The listing builds one solid part. Answer for the finished solid, in the listing's coordinates (mm). Face numbers are marked on the shaded views. A direction names the side the tool comes from. Give positions to 0.01 mm unless a question says otherwise; leave off trailing zeros. Order: outer loops, then holes, each group sorted by start corner. A loop starts at its lowest first (then second) coordinate and runs counter-clockwise, first axis right, second up. Notation, with made-up numbers: (57.25, 56) - (91.25, 56) arc R28 cw to (91.25, 90) - close; hole circle Ø4 at (-1.75, 30). An arc over 180 degrees is marked (long way). Write each question's results on one line, items separated by ' | '. Start each with the question number.
1. Section A-A (x = 22) is taken. Give the vertices of the cut face in (y, z).
2. Flat-ended cylindrical pins translate along their axes: pin 1 (8 mm diameter, centred on x = 33.5, y = 11, fed in from +Z); pin 2 (18.5 mm diameter, centred on x = 0, z = 0, fed in from -Y); pin 3 (1 mm diameter, centred on y = 4.5, z = -13, fed in from -X). Find the tip coordinate at first contact, or state that the pin passes through.
3. Which of the six approach directions +Z, -Z, +X, -X, +Y, -Y give full straight-line access (tool end or side, diameter ignored) to the marked faces 5 and 6?
4. Find the intervals of material crossed by L1, parallel to Z at x = 22, y = 14.5; L2, parallel to X at y = 10, z = -6.75; L3, parallel to Z at x = 0.5, y = 13.5, in increasing order.
5. Section B-B (y = 10) is taken. Give the vertices of the cut face in (x, z).
6. Section C-C (x = 31.7) is taken. Give the vertices of the cut face in (y, z), and give its area (3 significant figures).
7. Determine the mould class of the marked faces 1, 2, 3 and 4 for opening direction Z: released by +Z, released by -Z, zero draft, split by the parting line, or undercut.
8. Section D-D (z = 0) is taken. Give the vertices of the cut face in (x, y), and give its area (3 significant figures).
from build123d import *

# Parameters (mm, degrees)
DODANIE_WYCI_GNI_CIE1_DEPTH  = 20
ZAAWANSOWANYOTW_R1_START     = -11.5
ZAAWANSOWANYOTW_R1_OUTLINE_R = 5.5
ZAAWANSOWANYOTW_R1_DEPTH     = 23
ZAOKR_GLENIE3_R              = 2


# Read off the part's stored shape, not the designer's step: ZaawansowanyOtwór1
with BuildPart() as part:
    # Szkic1 → Dodanie-wyciągnięcie1 (new body)
    with BuildSketch(Plane(origin=(0, 0, 0), x_dir=(1, 0, 0), z_dir=(0, 1, 0))):
        with BuildLine():
            Line((12.109500403, 11.5), (39.7, 11.5))
            ThreePointArc((39.7, 11.5), (41.114213562, 10.914213562), (41.7, 9.5))
            Line((41.7, 9.5), (41.7, 4.5))
            ThreePointArc((41.7, 4.5), (41.114213562, 3.085786438), (39.7, 2.5))
            Line((39.7, 2.5), (13.774977314, 2.5))
            Line((13.774977314, 2.5), (12.939860896, 2.5))
            ThreePointArc((12.939860896, 2.5), (11.780953784, 2.869989477), (11.050830108, 3.843065693))
            ThreePointArc((11.050830108, 3.843065693), (-11.7, 0), (11.050830108, -3.843065693))
            ThreePointArc((11.050830108, -3.843065693), (11.780953784, -2.869989477), (12.939860896, -2.5))
            Line((12.939860896, -2.5), (13.774977314, -2.5))
            Line((13.774977314, -2.5), (39.7, -2.5))
            ThreePointArc((39.7, -2.5), (41.114213562, -3.085786438), (41.7, -4.5))
            Line((41.7, -4.5), (41.7, -9.5))
            ThreePointArc((41.7, -9.5), (41.114213562, -10.914213562), (39.7, -11.5))
            Line((39.7, -11.5), (12.109500403, -11.5))
            ThreePointArc((12.109500403, -11.5), (-16.7, 0), (12.109500403, 11.5))
        make_face()
    extrude(amount=DODANIE_WYCI_GNI_CIE1_DEPTH)

    # ZaawansowanyOtwór1 outline → ZaawansowanyOtwór1 (cut)
    with BuildSketch(Plane.XY.offset(ZAAWANSOWANYOTW_R1_START)):
        with Locations((31.7, 10)):
            Circle(ZAAWANSOWANYOTW_R1_OUTLINE_R)
    extrude(amount=ZAAWANSOWANYOTW_R1_DEPTH, mode=Mode.SUBTRACT)

    # Zaokrąglenie3
    zaokr_glenie3_edges = [part.edges().sort_by_distance(p)[0] for p in [
        (-16.7, 0, 0),
        (-16.7, 20, 0),
    ]]
    fillet(zaokr_glenie3_edges, radius=ZAOKR_GLENIE3_R)


solid = part.part
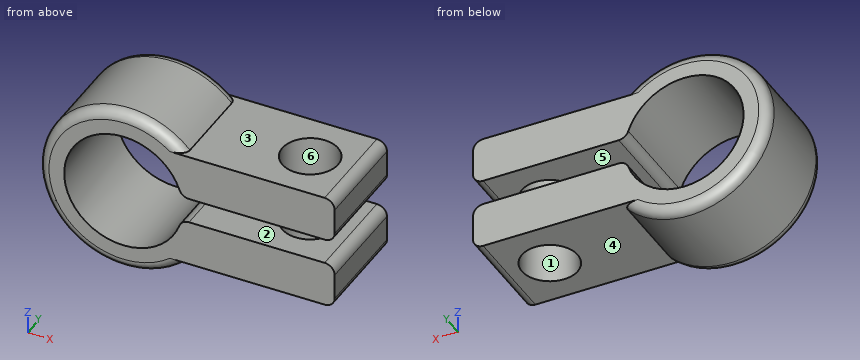
Reported:
1) outline: (0, -11.5) - (20, -11.5) - (20, -2.5) - (0, -2.5) - close; (0, 2.5) - (20, 2.5) - (20, 11.5) - (0, 11.5) - close
2) pin 1: z = 11.5 | pin 2: through | pin 3: x = -11.07
3) face 5: +X, +Y, -Y | face 6: +Z, -Z
4) L1: -11.5 to -2.5, 2.5 to 11.5 | L2: -15.28 to -9.56, 9.56 to 26.2, 37.2 to 41.7 | L3: -16.69 to -11.69, 11.69 to 16.69
5) outline: (11.05, -3.84) arc R11.7 cw (long way) to (11.05, 3.84) arc R2 ccw to (12.94, 2.5) - (26.2, 2.5) - (26.2, 11.5) - (12.11, 11.5) arc R16.7 ccw (long way) to (12.11, -11.5) - (26.2, -11.5) - (26.2, -2.5) - (12.94, -2.5) arc R2 ccw to start; (37.2, -11.5) - (39.7, -11.5) arc R2 ccw to (41.7, -9.5) - (41.7, -4.5) arc R2 ccw to (39.7, -2.5) - (37.2, -2.5) - close; (37.2, 2.5) - (39.7, 2.5) arc R2 ccw to (41.7, 4.5) - (41.7, 9.5) arc R2 ccw to (39.7, 11.5) - (37.2, 11.5) - close
6) outline: (0, -11.5) - (4.5, -11.5) - (4.5, -2.5) - (0, -2.5) - close; (0, 2.5) - (4.5, 2.5) - (4.5, 11.5) - (0, 11.5) - close; (15.5, -11.5) - (20, -11.5) - (20, -2.5) - (15.5, -2.5) - close; (15.5, 2.5) - (20, 2.5) - (20, 11.5) - (15.5, 11.5) - close | area: 162 mm²
7) face 1: zero draft | face 2: undercut | face 3: released by +Z | face 4: released by -Z
8) outline: (-16.7, 2) arc R2 ccw to (-14.7, 0) - (-11.7, 0) - (-11.7, 20) - (-14.7, 20) arc R2 ccw to (-16.7, 18) - close | area: 98.3 mm²
